CAD build for the part. Positions are in the model's coordinates, mm. A direction names the side the tool comes from. Give positions to 0.01 mm unless a question says otherwise; leave off trailing zeros. Order: outer loops, then holes, each group sorted by start corner. A loop starts at its lowest first (then second) coordinate and runs counter-clockwise, first axis right, second up. Notation, with made-up numbers: M -22,26 L 33,26 A15 ccw 33,35 Z; hole C 71.25,31 d9. An arc over 180 degrees is marked long. Put each result on its own line as item: value. Start each with the question number.
1) Two-plate mould, pull along Z, no slides. Class faces 1 (the face through (-110, 28, 4.804)), 2 (the face through (-119.2, 19.701, 3.7)), 3 (the face through (-120, 41.701, 6)): released by +Z, released by -Z, zero draft, split by the parting line, or undercut.
2) Cut at D-D (z = -5.75). Write the cut outline in (x, y), and give its area (3 significant figures).
3) Cut at C-C (y = 24.5). Write the cut outline in (x, z), and give its area (3 significant figures).
4) Cut at B-B (x = -123). Write the cut outline in (y, z).
5) Cut at A-A (y = 17.5). Write the cut outline in (x, z).
6) Pin check, flat tips, straight feed: pin 1 (8.5 mm diameter, centred on x = -130, y = 47.5, fed in from -Z); pin 2 (2.5 mm diameter, centred on x = -109.5, z = 7.5, fed in from -Y); pin 3 (7 mm diameter, centred on x = -119.23, z = 5, fed in from -Y); pin 4 (1.2 mm diameter, centred on x = -119.23, z = 5, fed in from -Y) (3 decimals). Stop position of each tip, or through.
7) Tool access for faces 4 (the face through (-111.72, 34.44, 3.96)), 5 (the face through (-124, 47, 0)), 6 (the face through (-129.787, 42.403, 4.93)), 7 (the face through (-122.16, 47.27, 5.65)): list every direction of +Z, -Z, +X, -X, +Y, -Y with a clear straight run to the whole face (end or side of a thin tool).
8) Drill centre lines: line 1 (Y direction, x = -131.25, z = 6.75); line 2 (Y direction, x = -117, z = 4.25); line 3 (X direction, y = 41, z = -3.5). Where is each one in solid material? Low to high. Write a range as [from, to].
```python
from build123d import *

# Parameters (mm, degrees)
CROQUIS1_R                = 2.5
SALIENTE_EXTRUIR1_DEPTH   = 10
CROQUIS2_R                = 1
CORTAR_EXTRUIR1_DEPTH     = 4
SALIENTE_EXTRUIR2_DEPTH   = 13.5
CROQUIS4_R                = 3
CORTAR_EXTRUIR2_DEPTH     = 1
SALIENTE_EXTRUIR3_START   = 6.5
CROQUIS6_R                = 3
SALIENTE_EXTRUIR3_DEPTH   = 6.5
CORTAR_EXTRUIR4_DEPTH     = 10
SALIENTE_EXTRUIR4_DEPTH   = 8.5
CORTAR_EXTRUIR5_START     = -5.196152423
CORTAR_EXTRUIR5_OUTLINE_W = 8
CORTAR_EXTRUIR5_OUTLINE_H = 10.5
CORTAR_EXTRUIR5_DEPTH     = 5.196152423
REDONDEO1_R               = 4


# Read off the part's stored shape, not the designer's step: Cortar-Extruir5
with BuildPart() as part:
    # Croquis1 → Saliente-Extruir1 (new body)
    with BuildSketch(Plane.XY):
        with BuildLine():
            Line((-106.231635218, 22.700651543), (-131.231635218, 22.700651543))
            Line((-131.231635218, 22.700651543), (-131.231635218, 20.200651543))
            ThreePointArc((-131.231635218, 20.200651543), (-135.231635218, 16.200651543), (-131.231635218, 12.200651543))
            Line((-131.231635218, 12.200651543), (-125.231635218, 12.200651543))
            Line((-125.231635218, 12.200651543), (-125.231635218, 18.700651543))
            Line((-125.231635218, 18.700651543), (-106.231635218, 18.700651543))
            Line((-106.231635218, 18.700651543), (-106.231635218, 22.700651543))
        make_face()
        with Locations((-131.231635218, 16.200651543)):
            Circle(CROQUIS1_R, mode=Mode.SUBTRACT)
    extrude(amount=SALIENTE_EXTRUIR1_DEPTH)

    # Croquis2 → Cortar-Extruir1 (cut)
    with BuildSketch(Plane.XZ.offset(-18.700651543)):
        with Locations(Location((-119.231635218, 5, 0), (0, 0, 270))):
            Circle(CROQUIS2_R)
        Polygon((-106.231635218, 0), (-106.231635218, 10), (-112.00513791, 0), align=None)
    extrude(amount=-CORTAR_EXTRUIR1_DEPTH, mode=Mode.SUBTRACT)

    # Croquis3 → Saliente-Extruir2 (add)
    with BuildSketch(Plane.XZ.offset(-18.700651543)):
        Polygon((-106.231635218, 10), (-108.231635218, 10), (-114.00513791, 0), (-112.00513791, 0), align=None)
    extrude(amount=-SALIENTE_EXTRUIR2_DEPTH)

    # Croquis4 → Cortar-Extruir2 (cut)
    with BuildSketch(Plane.XZ.offset(-18.700651543)):
        with Locations(Location((-119.231635218, 5, 0), (0, 0, 270))):
            Circle(CROQUIS4_R)
    extrude(amount=-CORTAR_EXTRUIR2_DEPTH, mode=Mode.SUBTRACT)

    # Croquis6 → Saliente-Extruir3 (add)
    with BuildSketch(Plane.XZ.offset(-18.700651543).offset(SALIENTE_EXTRUIR3_START)):
        Polygon((-125.231635218, 10), (-106.231635218, 10), (-112.00513791, 0), (-125.231635218, 0), align=None)
        with Locations(Location((-119.231635218, 5, 0), (0, 0, 270))):
            Circle(CROQUIS6_R, mode=Mode.SUBTRACT)
    extrude(amount=-SALIENTE_EXTRUIR3_DEPTH)

    # Croquis7 → Cortar-Extruir4 (cut)
    with BuildSketch(Plane.XY.offset(10)):
        Polygon((-106.231635218, 18.700651543), (-106.231635218, 12.200651543), (-125.231635218, 12.200651543), align=None)
    extrude(amount=-CORTAR_EXTRUIR4_DEPTH, mode=Mode.SUBTRACT)

    # Croquis8 → Saliente-Extruir4 (add)
    with BuildSketch(Plane(origin=(0, 0, 0), x_dir=(-1, 0, 0), z_dir=(0, 0, -1))):
        Polygon((112.00513791, 16.725505885), (112.00513791, 32.200651543), (114.00513791, 32.200651543), (114.00513791, 22.700651543), (114.00513791, 16.041295359), align=None)
    extrude(amount=SALIENTE_EXTRUIR4_DEPTH)

    # Simetría1: part across plane


with BuildPart() as part_1:
    add(part.part)
    add(part.part.mirror(Plane(origin=(0, 32.200651543, 0), x_dir=(0, 0, 1), z_dir=(0, -1, 0))))

    # Cortar-Extruir5 outline → Cortar-Extruir5 (cut)
    with BuildSketch(Plane.XY.offset(10).offset(CORTAR_EXTRUIR5_START)):
        with Locations((-109, 27.950651543)):
            Rectangle(CORTAR_EXTRUIR5_OUTLINE_W, CORTAR_EXTRUIR5_OUTLINE_H)
    extrude(amount=CORTAR_EXTRUIR5_DEPTH, mode=Mode.SUBTRACT)

    # Redondeo1
    # the kernel refuses this fillet: 4 mm, written as the material it takes off along each edge
    with BuildSketch(Plane(origin=(-131.231635218, 41.700651543, -9.270248109), x_dir=(1, 0, 0), z_dir=(0, 0, 1))) as redondeo1_piece_1:
        with BuildLine():
            CenterArc((3.708099244, 4), REDONDEO1_R, 202.024312837, 67.975687163)
            Line((0, 2.5), (-0.074161985, 2.47))
            ThreePointArc((-0.074161985, 2.47), (-0.08, 1.25), (-0.08, 0))
            Line((-0.08, 0), (0, -0.08))
            Line((0, -0.08), (3.708099244, -0.08))
            Line((3.708099244, -0.08), (3.708099244, 0))
        make_face()
    extrude(amount=28.540496218, mode=Mode.SUBTRACT)
    with BuildSketch(Plane(origin=(-131.231635218, 22.700651543, -9.270248109), x_dir=(0, -1, 0), z_dir=(0, 0, 1))) as redondeo1_piece_2:
        with BuildLine():
            CenterArc((4, 3.708099244), REDONDEO1_R, 180, 67.975687168)
            Line((0, 3.708099244), (-0.08, 3.708099244))
            Line((-0.08, 3.708099244), (-0.08, 0))
            Line((-0.08, 0), (0, -0.08))
            ThreePointArc((0, -0.08), (1.25, -0.08), (2.47, -0.074161985))
            Line((2.47, -0.074161985), (2.5, 0))
        make_face()
    extrude(amount=28.540496218, mode=Mode.SUBTRACT)


solid = part_1.part
```
Solution:
1. face 1: released by +Z
1. face 2: undercut
1. face 3: zero draft
2. outline: M -114.01,16.04 L -112.01,16.73 L -112.01,47.68 L -114.01,48.36 Z
2. area: 63.3 mm²
3. outline: M -114.01,-8.5 L -112.01,-8.5 L -112.01,0 L -109.23,4.8 L -111.23,4.8 L -114.01,0 Z
3. area: 26.6 mm²
4. outline: M 12.96,0 L 22.7,0 L 22.7,10 L 12.96,10 Z; M 41.7,0 L 51.44,0 L 51.44,10 L 41.7,10 Z
5. outline: M -135.01,0 L -133.37,0 L -133.37,10 L -135.01,10 Z; M -129.1,0 L -114.01,0 L -114.01,-8.5 L -112.01,-8.5 L -112.01,0 L -109.74,3.92 L -109.74,10 L -129.1,10 Z; hole C -119.23,5 d6
6. pin 1: z = 0
6. pin 2: y = 17.15
6. pin 3: y = 13.06
6. pin 4: through
7. face 4: +Z, -X
7. face 5: -Z, -X, +Y, -Y
7. face 6: +Z, -Z, -X
7. face 7: +Y
8. line 1: [12.2, 13.7], [18.7, 20.2], [44.2, 45.7], [50.7, 52.2]
8. line 2: [19.7, 22.7], [41.7, 44.7]
8. line 3: [-114.01, -112.01]
